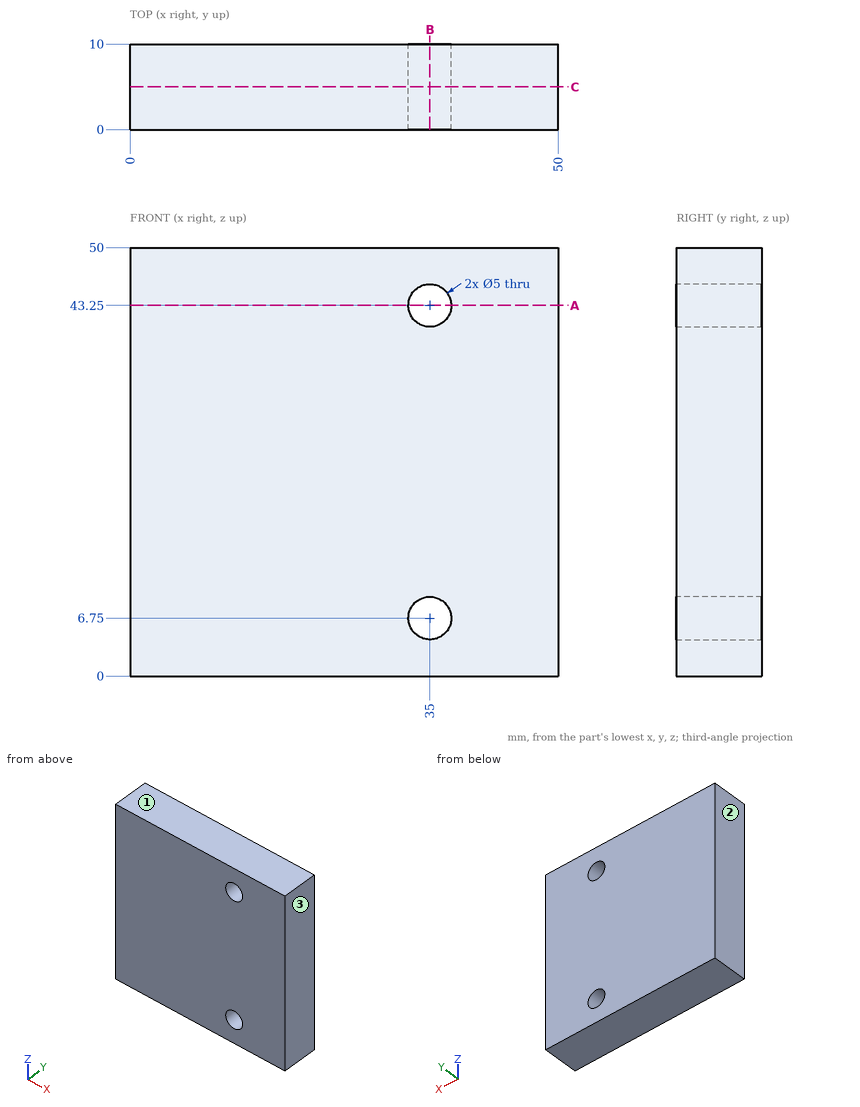
Geometry: see drawing. Coordinates: mm, zero at the bounding-box minimum. Give positions to 0.01 mm unless a question says otherwise; leave off trailing zeros. Write each loop counter-clockwise with the first axis right and the second up, starting at its lowest first coordinate (ties: lowest second). Pieces come first, ordered by that corner, then holes. Notation, with made-up numbers: (-4.75, -9.5) -> (45.25, -9.5) arc R17 cw to (45.25, 7.5) -> close; hole circle Ø7 at (-0.75, -2). An arc over 180 degrees is marked (long way). Use one line per item in the form item = value. Start each with the question number.
1) Section query B-B on x = 35. Return the cut outline in (y, z).
2) Section query C-C on y = 5. Return the cut outline in (x, z).
3) Ray query, probe 1 along X at (y, z) = (3, 43.25); probe 2 along X at (y, z) = (8.75, 6). Return the intervals inside material, ascending. Write a range as from..to.
4) Section query A-A on z = 43.25. Return the cut outline in (x, y).
5) Draft query along X for the marked faces 1, 2 and 3. Return one class per face: pulls with the +X half, pulls with the -X half, needs draft (parallel to the pull), parting line crosses it, or undercut.
Outcome:
q1.outline = (0, 0) -> (10, 0) -> (10, 4.25) -> (0, 4.25) -> close; (0, 9.25) -> (10, 9.25) -> (10, 40.75) -> (0, 40.75) -> close; (0, 45.75) -> (10, 45.75) -> (10, 50) -> (0, 50) -> close
q2.outline = (0, 0) -> (50, 0) -> (50, 50) -> (0, 50) -> close; hole circle Ø5 at (35, 6.75); hole circle Ø5 at (35, 43.25)
q3.probe_1 = 0..32.5, 37.5..50
q3.probe_2 = 0..32.62, 37.38..50
q4.outline = (0, 0) -> (32.5, 0) -> (32.5, 10) -> (0, 10) -> close; (37.5, 0) -> (50, 0) -> (50, 10) -> (37.5, 10) -> close
q5.face_1 = needs draft
q5.face_2 = pulls with the -X half
q5.face_3 = pulls with the +X half
